```python
from build123d import *

# Parameters (mm, degrees)
SKETCH1_W           = 140
SKETCH1_H           = 120
BOSS_EXTRUDE1_DEPTH = 8
SKETCH2_R           = 3.25
CUT_EXTRUDE1_DEPTH  = 93.54188241
CUT_EXTRUDE2_DEPTH  = 93.54188241
SKETCH5_W           = 50
SKETCH5_H           = 70
CUT_EXTRUDE3_DEPTH  = 93.54188241
FILLET2_R           = 5
FILLET3_R           = 5
SKETCH6_W           = 10.179307593
SKETCH6_H           = 120.009276429
SKETCH6_W_2         = 10
SKETCH6_H_2         = 120
CUT_EXTRUDE4_DEPTH  = 93.54188241
FILLET4_R           = 5


with BuildPart() as part:
    # Sketch1 → Boss-Extrude1 (new body)
    with BuildSketch(Plane.XY):
        Rectangle(SKETCH1_W, SKETCH1_H)
    extrude(amount=BOSS_EXTRUDE1_DEPTH)

    # Sketch2 → Cut-Extrude1 (cut, through all)
    with BuildSketch(Plane.XY.offset(8)):
        with Locations((-40, 20)):
            Circle(SKETCH2_R)
        with Locations((40, 20)):
            Circle(SKETCH2_R)
    extrude(amount=-CUT_EXTRUDE1_DEPTH, mode=Mode.SUBTRACT)

    # Sketch3 → Cut-Extrude2 (cut, through all)
    with BuildSketch(Plane.XY.offset(8)):
        with BuildLine():
            Line((-3.5, -49.9), (-3.5, -21.9))
            ThreePointArc((-3.5, -21.9), (0, -18.4), (3.5, -21.9))
            Line((3.5, -21.9), (3.5, -49.9))
            ThreePointArc((3.5, -49.9), (0, -53.4), (-3.5, -49.9))
        make_face()
    extrude(amount=-CUT_EXTRUDE2_DEPTH, mode=Mode.SUBTRACT)

    # Sketch5 → Cut-Extrude3 (cut, through all)
    with BuildSketch(Plane.XY.offset(8)):
        with Locations((0, 25)):
            Rectangle(SKETCH5_W, SKETCH5_H)
    extrude(amount=-CUT_EXTRUDE3_DEPTH, mode=Mode.SUBTRACT)

    # Fillet2
    fillet2_edges = [part.edges().sort_by_distance(p)[0] for p in [
        (-25, 25, 8),
        (25, 25, 8),
    ]]
    fillet(fillet2_edges, radius=FILLET2_R)

    # Fillet3
    # the kernel refuses this fillet: 5 mm, written as the material it takes off along each edge
    with BuildSketch(Plane(origin=(25, -10, 0), x_dir=(1, 0, 0), z_dir=(0, 1, 0)), Plane(origin=(-25, 71.456439237, 0), x_dir=(-1, 0, 0), z_dir=(0, -1, 0))) as fillet3_piece_1:
        with BuildLine():
            CenterArc((4.582575695, -5), FILLET3_R, 90, 66.421821522)
            Line((0, -3), (-0.091651514, -2.96))
            ThreePointArc((-0.091651514, -2.96), (-0.1, -1.5), (-0.1, 0))
            Line((-0.1, 0), (0, 0.1))
            Line((0, 0.1), (4.582575695, 0.1))
            Line((4.582575695, 0.1), (4.582575695, 0))
        make_face()
    extrude(amount=81.456439237, mode=Mode.SUBTRACT)

    # Sketch6 → Cut-Extrude4 (cut, through all)
    with BuildSketch(Plane.XY.offset(8)):
        with Locations((-64.910346203, 0.004638214)):
            Rectangle(SKETCH6_W, SKETCH6_H)
        with Locations((65, 0)):
            Rectangle(SKETCH6_W_2, SKETCH6_H_2)
    extrude(amount=-CUT_EXTRUDE4_DEPTH, mode=Mode.SUBTRACT)

    # Fillet4
    # the kernel refuses this fillet: 5 mm, written as the material it takes off along each edge
    with BuildSketch(Plane(origin=(60, 72.5, 0), x_dir=(0, 0, 1), z_dir=(0, -1, 0)), Plane(origin=(-59.820692407, -72.5, 8), x_dir=(1, 0, 0), z_dir=(0, 1, 0))) as fillet4_piece_1:
        with BuildLine():
            CenterArc((FILLET4_R, FILLET4_R), FILLET4_R, 180, 90)
            Line((0, FILLET4_R), (0, 0))
            Line((0, 0), (FILLET4_R, 0))
        make_face()
    extrude(amount=145, mode=Mode.SUBTRACT)
    with BuildSketch(Plane(origin=(60, -72.5, 8), x_dir=(-1, 0, 0), z_dir=(0, 1, 0)), Plane(origin=(-59.820692407, 72.5, 0), x_dir=(0, 0, 1), z_dir=(0, -1, 0))) as fillet4_piece_2:
        with BuildLine():
            CenterArc((FILLET4_R, -FILLET4_R), FILLET4_R, 90, 90)
            Line((0, -FILLET4_R), (0, 0))
            Line((0, 0), (FILLET4_R, 0))
        make_face()
    extrude(amount=145, mode=Mode.SUBTRACT)


solid = part.part
```
Geometry check sheet. Reference: the model listing, model coordinates, mm. A direction names the side the tool comes from. Round coordinates to 2 decimals unless told otherwise and drop trailing zeros. Loops run counter-clockwise (first coordinate to the right, second up) from the corner with the lowest first, then second, coordinate; pieces in that order, holes last. Notation, with made-up numbers: (86, -35.5) - (125, -35.5) arc R9 ccw to (125, -18.5) - close; hole circle Ø9 at (18.5, 3). An arc over 180 degrees is marked (long way). Use a Markdown table: item, result.
Q1. Go/stop test with flat-tipped pins: P1, Ø2.5, axis at x = 5.5, z = 5, coming from the +Y side; P2, Ø1, axis at y = -13.5, z = 6.5, coming from the +X side; P3, Ø2, axis at y = -25, z = 2.5, coming from the -X side. Record where each tip stops, or that it passes through.
Solutions:
| item | result |
|---|---|
| P1 | stops at y = -10 |
| P2 | stops at x = 59 |
| P3 | stops at x = -59.59 |
Q2. Cross-section at B-B on x = 40. Record the cut outline in (y, z).
Solutions:
| item | result |
|---|---|
| outline | (-60, 0) - (16.75, 0) - (16.75, 8) - (-60, 8) - close; (23.25, 0) - (60, 0) - (60, 8) - (23.25, 8) - close |
Q3. Access from +Z, -Z, +X, -X, +Y, -Y to the whole of each face (thin tool, end or side, straight path). Record for faces 5 (the cylindrical face through (0.1, -53.4, 4.1)), 6 (the cylindrical face through (26.878, 24.51, 0.795)), 7 (the flat face through (-1, -12, 8)), 8 (the cylindrical face through (27, 25, 7)).
Solutions:
| item | result |
|---|---|
| face 5 | +Z, -Z |
| face 6 | -Z, +Y |
| face 7 | +Z, +X, -X, +Y, -Y |
| face 8 | +Z, +Y |
Q4. Draft check along Y on faces 1 (the flat face through (-1, -60, 4)), 2 (the cylindrical face through (-27, 25, 7)), 3 (the cylindrical face through (43.002, 18.755, 4.056)), 4 (the flat face through (-3.5, -36, 4)). Enter one of: released by +Y, released by -Y, zero draft, split by the parting line, or undercut.
Solutions:
| item | result |
|---|---|
| face 1 | released by -Y |
| face 2 | zero draft |
| face 3 | undercut |
| face 4 | undercut |
Q5. Material ranges on line 1 (Y direction, x = 40, z = 3); line 2 (X direction, y = 17.5, z = 3.75); line 3 (Y direction, x = 39, z = 7.5), recorded low to high.
Solutions:
| item | result |
|---|---|
| line 1 | y = -60 to 16.75, 23.25 to 60 |
| line 2 | x = -59.66 to -42.08, -37.92 to -25.06, 25.06 to 37.92, 42.08 to 59.84 |
| line 3 | y = -60 to 16.91, 23.09 to 60 |
Q6. Cross-section at C-C on z = 1.25. Record the cut outline in (x, y), plus the area to 3 significant figures.
Solutions:
| item | result |
|---|---|
| outline | (-58.13, -60) - (58.31, -60) - (58.31, 60) - (26.28, 60) - (26.28, -10) - (-26.28, -10) - (-26.28, 60) - (-58.13, 60) - close; hole circle Ø6.5 at (-40, 20); hole (-3.5, -49.9) arc R3.5 ccw to (3.5, -49.9) - (3.5, -21.9) arc R3.5 ccw to (-3.5, -21.9) - close; hole circle Ø6.5 at (40, 20) |
| area | 9,990 mm2 |
Q7. Cross-section at A-A on y = 30.5. Record the cut outline in (x, z).
Solutions:
| item | result |
|---|---|
| outline | (-59.72, 4) arc R5 ccw to (-54.82, 0) - (-29.58, 0) arc R5 ccw to (-25, 3) arc R5 ccw to (-30, 8) - (-54.82, 8) arc R5 ccw to start; (25, 3) arc R5 ccw to (29.58, 0) - (55, 0) arc R5 ccw to (59.9, 4) arc R5 ccw to (55, 8) - (30, 8) arc R5 ccw to start |
Q8. Cross-section at D-D on y = -25.5. Record the cut outline in (x, z).
Solutions:
| item | result |
|---|---|
| outline | (-59.72, 4) arc R5 ccw to (-54.82, 0) - (-3.5, 0) - (-3.5, 8) - (-54.82, 8) arc R5 ccw to start; (3.5, 0) - (55, 0) arc R5 ccw to (59.9, 4) arc R5 ccw to (55, 8) - (3.5, 8) - close |
